```python
from build123d import *

# Parameters (mm, degrees)
SKETCH1_R                = 13.335
SKETCH1_R_2              = 10.795
BOSS_EXTRUDE1_DEPTH      = 21.336
SKETCH2_R                = 1.27
BOSS_EXTRUDE2_DEPTH      = 21.336
FILLET1_R                = 1.27
CIRPATTERN1_COUNT        = 4
FILLET1_OF_CIRPATTERN1_R = 1.27
SKETCH3_R                = 1.5875
BOSS_EXTRUDE3_DEPTH      = 3.175
FILLET2_R                = 1.27
SKETCH4_R                = 10.795
BOSS_EXTRUDE4_DEPTH      = 30.48
FILLET3_R                = 1.27
BOSS_EXTRUDE5_DEPTH      = 21.2852
SKETCH6_R                = 1.5875
BOSS_EXTRUDE6_DEPTH      = 6.985
SKETCH7_R                = 4.064
BOSS_EXTRUDE7_DEPTH      = 1.27
SKETCH8_R                = 12.7
SKETCH8_R_2              = 4.064
SKETCH8_R_3              = 3.81
BOSS_EXTRUDE10_DEPTH     = 4.572
SKETCH9_R                = 2.9972
BOSS_EXTRUDE12_DEPTH     = 1.778
SKETCH10_R               = 1.5875
BOSS_EXTRUDE13_DEPTH     = 25.4


with BuildPart() as part:
    # Sketch1 → Boss-Extrude1 (new body)
    with BuildSketch(Plane(origin=(0, 0, 0), x_dir=(0, 0, -1), z_dir=(1, 0, 0))):
        Circle(SKETCH1_R)
        Circle(SKETCH1_R_2, mode=Mode.SUBTRACT)
    extrude(amount=-BOSS_EXTRUDE1_DEPTH)

    # Sketch2 → Boss-Extrude2 (add)
    with BuildSketch(Plane(origin=(0, 0, 0), x_dir=(0, 0, -1), z_dir=(1, 0, 0))):
        with BuildLine():
            Line((8.944335097, -11.728214494), (7.934024936, -10.717904334))
            ThreePointArc((7.934024936, -10.717904334), (9.429268927, -9.429268927), (10.717904334, -7.934024936))
            Line((10.717904334, -7.934024936), (11.728214494, -8.944335097))
            ThreePointArc((11.728214494, -8.944335097), (11.728214494, -11.728214494), (8.944335097, -11.728214494))
        make_face()
        with Locations((10.336274795, -10.336274795)):
            Circle(SKETCH2_R, mode=Mode.SUBTRACT)
    boss_extrude2 = extrude(amount=-BOSS_EXTRUDE2_DEPTH)

    # Fillet1
    fillet1_edges = [part.edges().sort_by_distance(p)[0] for p in [
        (-10.668, -10.717904334, -7.934024936),
        (-10.668, -7.934024936, -10.717904334),
    ]]
    fillet(fillet1_edges, radius=FILLET1_R)

    # CirPattern1: Boss-Extrude2 ×4 about axis
    cirpattern1_axis = Axis((0, 0, 0), (1, 0, 0))
    for i in range(1, CIRPATTERN1_COUNT):
        add(boss_extrude2.rotate(cirpattern1_axis, i * 360 / CIRPATTERN1_COUNT))

    # Fillet1 of CirPattern1
    fillet1_of_cirpattern1_edges = [part.edges().sort_by_distance(p)[0] for p in [
        (-10.668, 7.934024936, -10.717904334),
        (-10.668, 10.717904334, -7.934024936),
        (-10.668, 10.717904334, 7.934024936),
        (-10.668, 7.934024936, 10.717904334),
        (-10.668, -7.934024936, 10.717904334),
        (-10.668, -10.717904334, 7.934024936),
    ]]
    fillet(fillet1_of_cirpattern1_edges, radius=FILLET1_OF_CIRPATTERN1_R)

    # Sketch3 → Boss-Extrude3 (add)
    # profile 1 of 2: a face of its own
    with BuildSketch(Plane(origin=(0, 0, 0), x_dir=(0, 0, -1), z_dir=(1, 0, 0))):
        with BuildLine():
            Line((-10.392294453, 2.921), (-4.677294453, 2.921))
            Line((-4.677294453, 2.921), (-4.677294453, -2.921))
            Line((-4.677294453, -2.921), (-10.392294453, -2.921))
            ThreePointArc((-10.392294453, -2.921), (-10.795, 0), (-10.392294453, 2.921))
        make_face()
        with Locations((-6.7945, 0)):
            Circle(SKETCH3_R, mode=Mode.SUBTRACT)
    # profile 2 of 2: a face of its own
    with BuildSketch(Plane(origin=(0, 0, 0), x_dir=(0, 0, -1), z_dir=(1, 0, 0))):
        with BuildLine():
            Line((10.392294453, 2.921), (4.677294453, 2.921))
            Line((4.677294453, 2.921), (4.677294453, -2.921))
            Line((4.677294453, -2.921), (10.392294453, -2.921))
            ThreePointArc((10.392294453, -2.921), (10.795, 0), (10.392294453, 2.921))
        make_face()
        with Locations((6.7945, 0)):
            Circle(SKETCH3_R, mode=Mode.SUBTRACT)
    extrude(amount=-BOSS_EXTRUDE3_DEPTH)

    # Fillet2
    fillet2_edges = [part.edges().sort_by_distance(p)[0] for p in [
        (-1.5875, -2.921, -4.677294453),
        (-1.5875, 2.921, -4.677294453),
        (-1.5875, 2.921, 4.677294453),
        (-1.5875, -2.921, 4.677294453),
    ]]
    fillet(fillet2_edges, radius=FILLET2_R)

    # Sketch4 → Boss-Extrude4 (add)
    with BuildSketch(Plane.ZY.offset(3.175)):
        with Locations(Location((0, 0, 0), (0, 0, 180))):
            Circle(SKETCH4_R)
    extrude(amount=BOSS_EXTRUDE4_DEPTH)

    # Fillet3
    fillet3_edges = [part.edges().sort_by_distance(p)[0] for p in [
        (-33.655, 0, 10.795),
    ]]
    fillet(fillet3_edges, radius=FILLET3_R)

    # Sketch5 → Boss-Extrude5 (add)
    with BuildSketch(Plane(origin=(0, 0, 0), x_dir=(0, 0, -1), z_dir=(1, 0, 0))):
        with BuildLine():
            Line((-11.919383507, 11.506214561), (-5.969, 19.558))
            Line((-5.969, 19.558), (-5.969, 29.718))
            Line((-5.969, 29.718), (5.969, 29.718))
            Line((5.969, 29.718), (5.969, 19.558))
            Line((5.969, 19.558), (11.919383507, 11.506214561))
            ThreePointArc((11.919383507, 11.506214561), (10.482758209, 12.299317041), (8.944335097, 11.728214494))
            Line((8.944335097, 11.728214494), (8.678267418, 11.462146816))
            ThreePointArc((8.678267418, 11.462146816), (7.921930715, 11.098101014), (7.10369904, 11.285374825))
            ThreePointArc((7.10369904, 11.285374825), (0, 13.335), (-7.10369904, 11.285374825))
            ThreePointArc((-7.10369904, 11.285374825), (-7.921930715, 11.098101014), (-8.678267418, 11.462146816))
            Line((-8.678267418, 11.462146816), (-8.944335097, 11.728214494))
            ThreePointArc((-8.944335097, 11.728214494), (-10.482758209, 12.299317041), (-11.919383507, 11.506214561))
        make_face()
    extrude(amount=-BOSS_EXTRUDE5_DEPTH)

    # Sketch6 → Boss-Extrude6 (add)
    with BuildSketch(Plane(origin=(-3.175, 0, 0), x_dir=(0, 0, -1), z_dir=(1, 0, 0))):
        with Locations(Location((0, 0, 0), (0, 0, 180))):
            Circle(SKETCH6_R)
    extrude(amount=BOSS_EXTRUDE6_DEPTH)

    # Sketch7 → Boss-Extrude7 (add)
    with BuildSketch(Plane(origin=(0, 0, 0), x_dir=(0, 0, -1), z_dir=(1, 0, 0))):
        with Locations((0, 16.256)):
            Circle(SKETCH7_R)
    extrude(amount=BOSS_EXTRUDE7_DEPTH)

    # Sketch8 → Boss-Extrude10 (add)
    # profile 1 of 3: a face of its own
    with BuildSketch(Plane(origin=(1.27, 0, 0), x_dir=(0, 0, -1), z_dir=(1, 0, 0))):
        with Locations((0, 16.256)):
            Circle(SKETCH8_R)
        with Locations((0, 16.256)):
            Circle(SKETCH8_R_2, mode=Mode.SUBTRACT)
    # profile 2 of 3: a face of its own
    with BuildSketch(Plane(origin=(1.27, 0, 0), x_dir=(0, 0, -1), z_dir=(1, 0, 0))):
        with Locations((0, 16.256)):
            Circle(SKETCH8_R_2)
    # profile 3 of 3: a face of its own
    with BuildSketch(Plane(origin=(1.27, 0, 0), x_dir=(0, 0, -1), z_dir=(1, 0, 0))):
        Circle(SKETCH8_R_3)
    extrude(amount=BOSS_EXTRUDE10_DEPTH)

    # Sketch9 → Boss-Extrude12 (add)
    with BuildSketch(Plane(origin=(5.842, 0, 0), x_dir=(0, 0, -1), z_dir=(1, 0, 0))):
        with Locations((0, 16.256)):
            Circle(SKETCH9_R)
    extrude(amount=BOSS_EXTRUDE12_DEPTH)

    # Sketch10 → Boss-Extrude13 (add)
    with BuildSketch(Plane(origin=(7.62, 0, 0), x_dir=(0, 0, -1), z_dir=(1, 0, 0))):
        with Locations((0, 16.256)):
            Circle(SKETCH10_R)
    extrude(amount=BOSS_EXTRUDE13_DEPTH)


solid = part.part
```
Could you check a few things on this model? Use its own coordinates, in mm. A direction names the side the tool comes from. Round coordinates to 2 decimals unless told otherwise and drop trailing zeros. Order: outer loops, then holes, each group sorted by start corner. A loop starts at its lowest first (then second) coordinate and runs counter-clockwise, first axis right, second up. Notation, with made-up numbers: M -17,12.5 L 19,12.5 A21 ccw 19,46.5 Z; hole C -38.75,-26.5 d2. An arc over 180 degrees is marked long. One line per question, with ' | ' between items. Start each with the question number.
(1) Thinking about a two-plate mould opening in X: for faces 5 (the face through (0, 13, 3)), 6 (the face through (33.02, 16, 0)), 7 (the face through (-1.57, 0.48, 5.28)), which applies, +X half, -X half, draft (parallel to the pull), parting line (faces both ways), or undercut?
(2) Suppose I cut it at D-D on x = 13. List the corners of the cut face in (y, z) for me (1 decimal).
(3) For P1, Ø3, axis at x = -5.5, y = 24, coming from the +Z side; P2, Ø2, axis at x = 0, z = -10, coming from the -Y side; P3, Ø3, axis at y = 10.34, z = 10.34, coming from the -X side; P4, Ø2, axis at y = -10.34, z = -10.34, coming from the -X side, each with a flat end and sliding along its axis, tell me the tip position at first contact or that it passes through.
(4) For faces 1 (the face through (-1.57, -0.61, -8.26)), 2 (the face through (-10.49, 15.59, -8.9)), 3 (the face through (-26.783, -7.296, 7.956)), 4 (the face through (-10, 25, 5.969)), which set-ups out of +Z, -Z, +X, -X, +Y, -Y let a thin tool reach every point of the face, with its end or its side?
(5) Please list where these lines run through material, in increasing order: line 1 along X through (y, z) = (26, 0.5); line 2 along Y through (x, z) = (-14.5, -12); line 3 along Y through (x, z) = (-12.5, -9.25).
(6) Suppose I cut it at C-C on x = -25.5. List the corners of the cut face in (y, z) for me (3 decimals).
(7) Suppose I cut it at A-A on x = -17. Count the separate pieces of the cut face and the enclosed holes in it, then the cut area to 3 significant figures.
Geometry results:
1) face 5: undercut | face 6: +X half | face 7: draft
2) outline: C 16.3,0 d3.2
3) P1: z = 5.97 | P2: y = -12.3 | P3: x = -21.34 | P4: through
4) face 1: +X | face 2: -Z, -X, +Y | face 3: -X | face 4: +Z, -X, +Y
5) line 1: -21.29 to 0, 1.27 to 5.84 | line 2: -11.39 to -9.28, -5.82 to 5.82, 9.28 to 11.39 | line 3: -11.98 to -10.99, -9.68 to 9.68, 10.99 to 15.12
6) outline: C 0,0 d21.59
7) separate pieces: 1 | enclosed holes: 4 | area: 832 mm²
